The model under review builds one solid part; all positions refer to its coordinate system, in mm. A direction names the side the tool comes from. Coordinates: 2 decimals unless noted, no trailing zeros. Loops run counter-clockwise (first coordinate to the right, second up) from the corner with the lowest first, then second, coordinate; pieces in that order, holes last. Notation, with made-up numbers: M 8.5,-38.5 L 56.5,-38.5 A27 cw 56.5,-10.5 Z; hole C -11.75,38 d3. An arc over 180 degrees is marked long. Use CSV: the item, a comma, the result in double quotes. Start each with the question number.
1. Add section C-C, the plane z = 0.7. Write out the cut boundary in (x, y).
2. Tool access review of faces 1 (the cylindrical face through (-1.53, -6.87, 3.75)), 2 (the cylindrical face through (-12, 0, 2)): name each direction out of +Z, -Z, +X, -X, +Y, -Y from which nothing blocks a thin tool from reaching the whole face with its end or side.
3. For L1, parallel to Z at x = 6.5, y = -3.5; L2, parallel to X at y = 0.25, z = 1.7; L3, parallel to X at y = -4.5, z = 3.45, list the stretches that pass through material, from the lowest coordinate up.
4. Add section A-A, the plane y = 0. Write out the cut boundary in (x, z), then the cut area to 3 significant figures.
5. Add section B-B, the plane x = 2.5. Write out the cut boundary in (y, z), then the cut area to 3 significant figures.
from build123d import *

# Parameters (mm, degrees)
BOSS_EXTRUDE1_DEPTH = 3.5
SKETCH2_R           = 7.036998645
BOSS_EXTRUDE2_DEPTH = 0.5
FILLET1_R           = 0.2


with BuildPart() as part:
    # Sketch1 → Boss-Extrude1 (new body)
    with BuildSketch(Plane.XY):
        with BuildLine():
            Line((-4.5, -7.5), (4.5, -7.5))
            ThreePointArc((4.5, -7.5), (12, 0), (4.5, 7.5))
            Line((4.5, 7.5), (-4.5, 7.5))
            ThreePointArc((-4.5, 7.5), (-12, 0), (-4.5, -7.5))
        make_face()
    extrude(amount=BOSS_EXTRUDE1_DEPTH)

    # Sketch2 → Boss-Extrude2 (add)
    with BuildSketch(Plane.XY.offset(3.5)):
        Circle(SKETCH2_R)
    extrude(amount=BOSS_EXTRUDE2_DEPTH)

    # Fillet1
    fillet1_edges = [part.edges().sort_by_distance(p)[0] for p in [
        (-12, 0, 3.5),
        (0, -7.5, 3.5),
        (12, 0, 3.5),
        (0, -7.5, 0),
        (-12, 0, 0),
        (0, 7.5, 0),
        (12, 0, 0),
        (0, 7.5, 3.5),
    ]]
    fillet(fillet1_edges, radius=FILLET1_R)


solid = part.part
Computed:
1,outline,"M -4.5,-7.5 L 4.5,-7.5 A7.5 ccw 4.5,7.5 L -4.5,7.5 A7.5 ccw Z"
2,face 1,"+Z"
2,face 2,"+Z, -Z, -X"
3,L1,"z = 0 to 3.5"
3,L2,"x = -12 to 12"
3,L3,"x = -10.42 to 10.42"
4,outline,"M -12,0.2 A0.2 ccw -11.8,0 L 11.8,0 A0.2 ccw 12,0.2 L 12,3.3 A0.2 ccw 11.8,3.5 L 7.04,3.5 L 7.04,4 L -7.04,4 L -7.04,3.5 L -11.8,3.5 A0.2 ccw -12,3.3 Z"
4,area,"91.0 mm^2"
5,outline,"M -7.5,0.2 A0.2 ccw -7.3,0 L 7.3,0 A0.2 ccw 7.5,0.2 L 7.5,3.3 A0.2 ccw 7.3,3.5 L 6.58,3.5 L 6.58,4 L -6.58,4 L -6.58,3.5 L -7.3,3.5 A0.2 ccw -7.5,3.3 Z"
5,area,"59.0 mm^2"
